from build123d import *

# Parameters (mm, degrees)
SKETCH2_R           = 5
SKETCH2_R_2         = 1.5
BOSS_EXTRUDE1_DEPTH = 3
FILLET1_R           = 3
SKETCH3_R           = 8
SKETCH3_R_2         = 5
BOSS_EXTRUDE2_DEPTH = 8.04


with BuildPart() as part:
    # Sketch2 → Boss-Extrude1 (new body)
    with BuildSketch(Plane(origin=(0, 0, 0), x_dir=(1, 0, 0), z_dir=(0, 1, 0))):
        with BuildLine():
            Line((30, 4), (30, 12))
            Line((30, 12), (18.98340249, 14.937759336))
            ThreePointArc((18.98340249, 14.937759336), (15, 16), (11.01659751, 14.937759336))
            Line((11.01659751, 14.937759336), (0, 12))
            Line((0, 12), (0, 4))
            Line((0, 4), (11.01659751, 1.062240664))
            ThreePointArc((11.01659751, 1.062240664), (15, 0), (18.98340249, 1.062240664))
            Line((18.98340249, 1.062240664), (30, 4))
        make_face()
        with Locations(Location((15, 8, 0), (0, 0, 270))):
            Circle(SKETCH2_R, mode=Mode.SUBTRACT)
        with Locations(Location((26.25, 8, 0), (0, 0, 270))):
            Circle(SKETCH2_R_2, mode=Mode.SUBTRACT)
        with Locations(Location((3.75, 8, 0), (0, 0, 90))):
            Circle(SKETCH2_R_2, mode=Mode.SUBTRACT)
    extrude(amount=BOSS_EXTRUDE1_DEPTH)

    # Fillet1
    fillet1_edges = [part.edges().sort_by_distance(p)[0] for p in [
        (0, 1.5, -4),
        (0, 1.5, -12),
        (30, 1.5, -12),
        (30, 1.5, -4),
    ]]
    fillet(fillet1_edges, radius=FILLET1_R)

    # Sketch3 → Boss-Extrude2 (add)
    with BuildSketch(Plane(origin=(0, 3, 0), x_dir=(1, 0, 0), z_dir=(0, 1, 0))):
        with Locations(Location((15, 8, 0), (0, 0, 60.137165644))):
            Circle(SKETCH3_R)
        with Locations(Location((15, 8, 0), (0, 0, 270))):
            Circle(SKETCH3_R_2, mode=Mode.SUBTRACT)
    extrude(amount=BOSS_EXTRUDE2_DEPTH)


solid = part.part
The model under review builds one solid part; all positions refer to its coordinate system, in mm. Coordinates: 2 decimals unless noted, no trailing zeros. Write each loop counter-clockwise with the first axis right and the second up, starting at its lowest first coordinate (ties: lowest second). Pieces come first, ordered by that corner, then holes. Notation, with made-up numbers: (-39.5, -10) -> (-23.5, -10) arc R8 ccw to (-23.5, 1) -> close; hole circle Ø4 at (48.5, 57). An arc over 180 degrees is marked (long way). Answer in a Markdown table with one row per item.
1. We need section B-B, the plane z = -8. State the section outline as (x, y) points, and give its area (3 significant figures).
Answers below:
| item | result |
|---|---|
| outline | (0, 0) -> (2.25, 0) -> (2.25, 3) -> (0, 3) -> close; (5.25, 0) -> (10, 0) -> (10, 11.04) -> (7, 11.04) -> (7, 3) -> (5.25, 3) -> close; (20, 0) -> (24.75, 0) -> (24.75, 3) -> (23, 3) -> (23, 11.04) -> (20, 11.04) -> close; (27.75, 0) -> (30, 0) -> (30, 3) -> (27.75, 3) -> close |
| area | 90.2 mm^2 |
2. Wall thickness on probe 1 along X at (y, z) = (1.8, -8); probe 2 along X at (y, z) = (4.25, -8); probe 3 along Y at (x, z) = (27.75, -5): over which ranges is each line inside the solid? List them lowest first. Write a range as [from, to].
Answers below:
| item | result |
|---|---|
| probe 1 | x = [0, 2.25], [5.25, 10], [20, 24.75], [27.75, 30] |
| probe 2 | x = [7, 10], [20, 23] |
| probe 3 | y = [0, 3] |
3. We need section A-A, the plane x = 26.25. State the section outline as (y, z) points, and give its area (3 significant figures).
Answers below:
| item | result |
|---|---|
| outline | (0, -13) -> (3, -13) -> (3, -9.5) -> (0, -9.5) -> close; (0, -6.5) -> (3, -6.5) -> (3, -3) -> (0, -3) -> close |
| area | 21.0 mm^2 |
4. Draft analysis for pull direction X (two halves, no side actions). For faces 1 (the flat face through (23.32, 1.48, -2.22)), 2 (the flat face through (19.5, 11.04, -5.3)), 3 (the cylindrical face through (2.74, 1.48, -6.89)), state which applies: +X half, -X half, draft (parallel to the pull), parting line (faces both ways), or undercut.
Answers below:
| item | result |
|---|---|
| face 1 | +X half |
| face 2 | draft |
| face 3 | undercut |
5. We need section C-C, the plane y = 1. State the section outline as (x, z) points, and give its area (3 significant figures).
Answers below:
| item | result |
|---|---|
| outline | (0, -9.7) arc R3 ccw to (2.23, -12.59) -> (11.02, -14.94) arc R8 ccw to (18.98, -14.94) -> (27.77, -12.59) arc R3 ccw to (30, -9.7) -> (30, -6.3) arc R3 ccw to (27.77, -3.41) -> (18.98, -1.06) arc R8 ccw to (11.02, -1.06) -> (2.23, -3.41) arc R3 ccw to (0, -6.3) -> close; hole circle Ø3 at (3.75, -8); hole circle Ø10 at (15, -8); hole circle Ø3 at (26.25, -8) |
| area | 266 mm^2 |
6. Clearance check with flat-ended pins moving along their axes: pin 1 Ø3 at (x, y) = (20.5, 9) entering from +Z; pin 2 Ø1 at (y, z) = (8, -11) entering from -X; pin 3 Ø4 at (x, y) = (23.5, 6) entering from +Z. State where each tip first meets the part, or that it passes through.
Answers below:
| item | result |
|---|---|
| pin 1 | stops at z = -1.07 |
| pin 2 | stops at x = 7.4 |
| pin 3 | stops at z = -3.34 |
7. We need section D-D, the plane x = 15. State the section outline as (y, z) points, and give its area (3 significant figures).
Answers below:
| item | result |
|---|---|
| outline | (0, -16) -> (11.04, -16) -> (11.04, -13) -> (0, -13) -> close; (0, -3) -> (11.04, -3) -> (11.04, 0) -> (0, 0) -> close |
| area | 66.2 mm^2 |
